For this review, take the finished solid that the model builds, in its own axes (mm). Round coordinates to 2 decimals unless told otherwise and drop trailing zeros. Write each loop counter-clockwise with the first axis right and the second up, starting at its lowest first coordinate (ties: lowest second). Pieces come first, ordered by that corner, then holes. Notation, with made-up numbers: M -5.75,65.25 L 4.25,65.25 A35 cw 4.25,104.25 Z; hole C 16.5,-28.75 d1. An arc over 180 degrees is marked long. Answer in a Markdown table with one row per item.
```python
from build123d import *


with BuildPart() as part:
    # Croquis1 → Revolución1 (revolve)
    with BuildSketch(Plane(origin=(0, 0, 0), x_dir=(1, 0, 0), z_dir=(0, 1, 0)), mode=Mode.PRIVATE) as revoluci_n1_sk:
        with BuildLine():
            Line((1.5, 4.25), (1.5, 4.75))
            ThreePointArc((1.5, 4.75), (1.426776695, 4.926776695), (1.25, 5))
            Line((1.25, 5), (-1.25, 5))
            ThreePointArc((-1.25, 5), (-1.426776695, 4.926776695), (-1.5, 4.75))
            Line((-1.5, 4.75), (-1.5, 4.25))
            ThreePointArc((-1.5, 4.25), (-1.426776695, 4.073223305), (-1.25, 4))
            Line((-1.25, 4), (1.25, 4))
            ThreePointArc((1.25, 4), (1.426776695, 4.073223305), (1.5, 4.25))
        make_face()
    revolve(revoluci_n1_sk.sketch.rotate(Axis((0, 0, 0), (1, 0, 0)), 180), axis=Axis((0, 0, 0), (1, 0, 0)))


solid = part.part
```
Q1. Insertion check: P1, Ø1.5, axis at y = 2.5, z = 1, coming from the -X side. The pin has a flat end and moves straight along its axis. Give the tip position at first contact, or say it passes through.
Found:
| item | result |
|---|---|
| P1 | through |
Q2. Mouldability with a two-part tool opening along Z and no side actions: class faces 1 (the face through (0, 0, -5)), 2 (the face through (-1.5, 2, -4)), 3 (the face through (0.018, 3.905, -0.867)) as +Z half, -Z half, draft (parallel to the pull), parting line (faces both ways), or undercut.
Found:
| item | result |
|---|---|
| face 1 | parting line |
| face 2 | draft |
| face 3 | undercut |
Q3. Take a section at C-C (x = -0.45). State the section outline as (y, z) points, then the cut area to 3 significant figures.
Found:
| item | result |
|---|---|
| outline | C 0,0 d10; hole C 0,0 d8 |
| area | 28.3 mm² |
Q4. For probe 1 along Y at (x, z) = (-0.45, 0); probe 2 along Y at (x, z) = (1.4, 3); probe 3 along Z at (x, y) = (-0.2, -3), list the stretches that pass through material, from the lowest coordinate up.
Found:
| item | result |
|---|---|
| probe 1 | -5 to -4, 4 to 5 |
| probe 2 | -3.94 to -2.72, 2.72 to 3.94 |
| probe 3 | -4 to -2.65, 2.65 to 4 |
Q5. Take a section at A-A (y = 0). State the section outline as (x, z) points.
Found:
| item | result |
|---|---|
| outline | M -1.5,-4.75 A0.25 ccw -1.25,-5 L 1.25,-5 A0.25 ccw 1.5,-4.75 L 1.5,-4.25 A0.25 ccw 1.25,-4 L -1.25,-4 A0.25 ccw -1.5,-4.25 Z; M -1.5,4.25 A0.25 ccw -1.25,4 L 1.25,4 A0.25 ccw 1.5,4.25 L 1.5,4.75 A0.25 ccw 1.25,5 L -1.25,5 A0.25 ccw -1.5,4.75 Z |
